For this review, use the dimensioned drawing (mm, ordinates from the lowest corner) and the shaded views. A direction names the side the tool comes from. Coordinates: 2 decimals unless noted, no trailing zeros. Order: outer loops, then holes, each group sorted by start corner. A loop starts at its lowest first (then second) coordinate and runs counter-clockwise, first axis right, second up. Notation, with made-up numbers: M 57.25,54.5 L 116.25,54.5 A23 cw 116.25,75.5 Z; hole C -37,5 d1. An arc over 180 degrees is marked long. Answer in a Markdown table with one row per item.
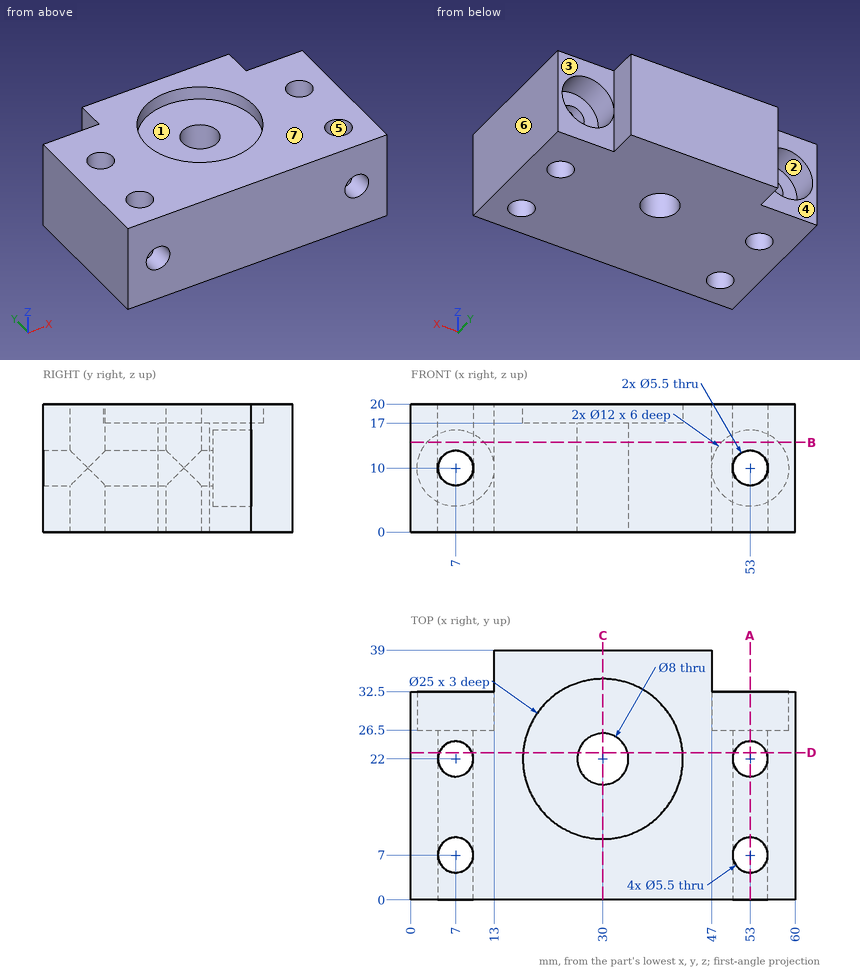
(1) Add section D-D, the plane y = 23. Give the boundary of the cut face in (x, z).
Return value:
| item | result |
|---|---|
| outline | M 0,0 L 4.44,0 L 4.44,9 A2.75 cw 4.44,11 L 4.44,20 L 0,20 Z; M 9.56,0 L 26.13,0 L 26.13,17 L 17.54,17 L 17.54,20 L 9.56,20 L 9.56,11 A2.75 cw 9.56,9 Z; M 33.87,0 L 50.44,0 L 50.44,9 A2.75 cw 50.44,11 L 50.44,20 L 42.46,20 L 42.46,17 L 33.87,17 Z; M 55.56,0 L 60,0 L 60,20 L 55.56,20 L 55.56,11 A2.75 cw 55.56,9 Z |
(2) For line 1 along X through (y, z) = (14, 10); line 2 along Y through (x, z) = (53, 15.5); line 3 along Y through (x, z) = (30, 17.8), list the stretches that pass through material, from the lowest coordinate up. Write a range as from..to.
Return value:
| item | result |
|---|---|
| line 1 | x = 0..4.25, 9.75..50.25, 55.75..60 |
| line 2 | y = 0..4.25, 9.75..19.25, 24.75..26.5 |
| line 3 | y = 0..9.5, 34.5..39 |
(3) Insertion check: pin 1 Ø9.5 at (x, z) = (54, 8.5) entering from +Y; pin 2 Ø3 at (y, z) = (36, 8) entering from +X; pin 3 Ø7 at (x, z) = (7, 10) entering from +Y. Each pin has a flat end and moves straight along its axis. Give the tip position at first contact, or say it passes through.
Return value:
| item | result |
|---|---|
| pin 1 | stops at y = 32.5 |
| pin 2 | stops at x = 47 |
| pin 3 | stops at y = 26.5 |
(4) Add section C-C, the plane x = 30. Give the boundary of the cut face in (y, z), and give its area (3 significant figures).
Return value:
| item | result |
|---|---|
| outline | M 0,0 L 18,0 L 18,17 L 9.5,17 L 9.5,20 L 0,20 Z; M 26,0 L 39,0 L 39,20 L 34.5,20 L 34.5,17 L 26,17 Z |
| area | 569 mm2 |
(5) For the marked faces 1, 2, 3 and 4, list the 3-axis set-ups (+Z, -Z, +X, -X, +Y, -Y) from which the entire face can be reached by the end or side of a thin tool; tool diameter is ignored.
Return value:
| item | result |
|---|---|
| face 1 | +Z |
| face 2 | +Y |
| face 3 | +Z, -Z, +X, +Y |
| face 4 | +Z, -Z, -X, +Y |
(6) Add section A-A, the plane x = 53. Give the boundary of the cut face in (y, z).
Return value:
| item | result |
|---|---|
| outline | M 0,0 L 4.25,0 L 4.25,7.25 L 0,7.25 Z; M 0,12.75 L 4.25,12.75 L 4.25,20 L 0,20 Z; M 9.75,0 L 19.25,0 L 19.25,7.25 L 9.75,7.25 Z; M 9.75,12.75 L 19.25,12.75 L 19.25,20 L 9.75,20 Z; M 24.75,0 L 32.5,0 L 32.5,4 L 26.5,4 L 26.5,7.25 L 24.75,7.25 Z; M 24.75,12.75 L 26.5,12.75 L 26.5,16 L 32.5,16 L 32.5,20 L 24.75,20 Z |
(7) Draft analysis for pull direction X (two halves, no side actions). For the marked faces 5, 6 and 7, state which applies: pulls with the +X half, pulls with the -X half, needs draft (parallel to the pull), parting line crosses it, or undercut.
Return value:
| item | result |
|---|---|
| face 5 | undercut |
| face 6 | pulls with the +X half |
| face 7 | needs draft |
(8) Add section B-B, the plane z = 14. Give the boundary of the cut face in (x, y).
Return value:
| item | result |
|---|---|
| outline | M 0,0 L 60,0 L 60,32.5 L 57.47,32.5 L 57.47,26.5 L 48.53,26.5 L 48.53,32.5 L 47,32.5 L 47,39 L 13,39 L 13,32.5 L 11.47,32.5 L 11.47,26.5 L 2.53,26.5 L 2.53,32.5 L 0,32.5 Z; hole C 7,7 d5.5; hole C 7,22 d5.5; hole C 30,22 d8; hole C 53,7 d5.5; hole C 53,22 d5.5 |
